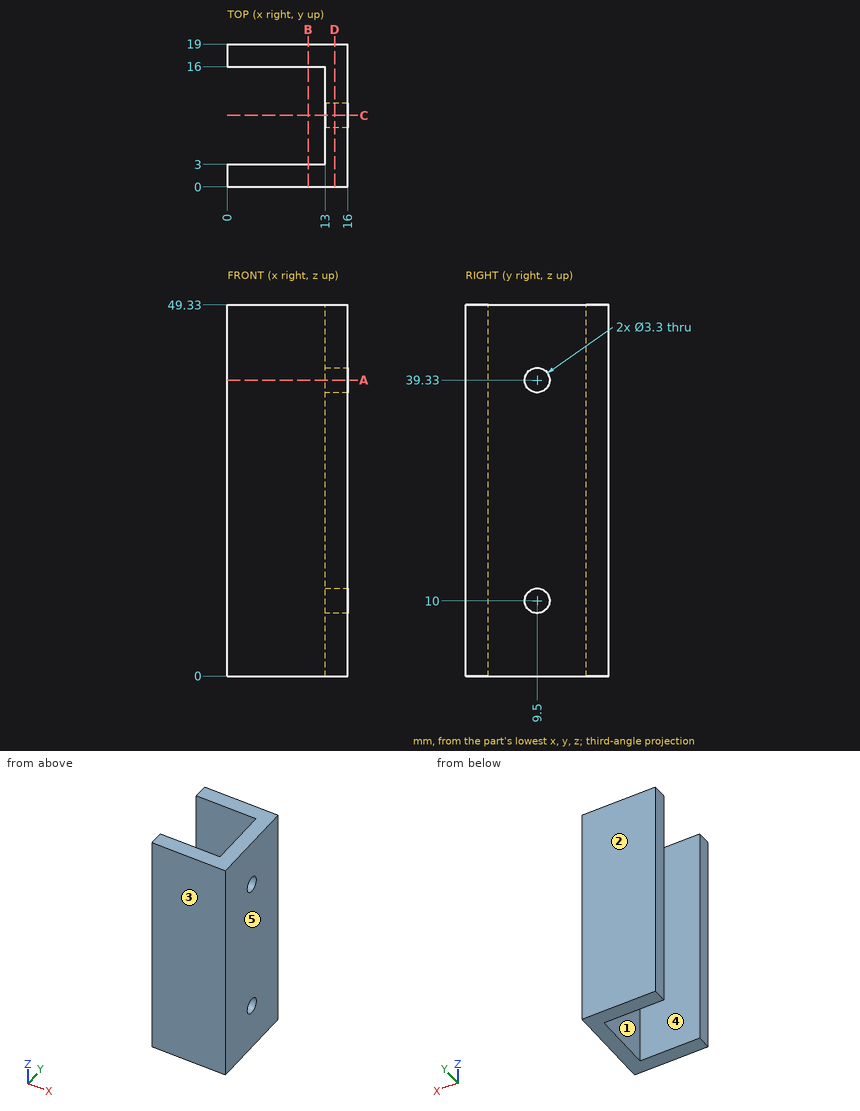
Can you work these out from the drawing? Everything is in mm from the part's minimum corner. A direction names the side the tool comes from. Round coordinates to 2 decimals unless told otherwise and drop trailing zeros. Order: outer loops, then holes, each group sorted by start corner. A loop starts at its lowest first (then second) coordinate and runs counter-clockwise, first axis right, second up. Notation, with made-up numbers: M 27,-37 L 59,-37 A27 cw 59,-15 Z; hole C -25,58.5 d11. An arc over 180 degrees is marked long. One line per question, with ' | ' between items.
1) I want a section at D-D, the plane x = 14.25. Write out the boundary of the cut face in (y, z).
Working result:
outline: M 0,0 L 19,0 L 19,49.33 L 0,49.33 Z; hole C 9.5,10 d3.3; hole C 9.5,39.33 d3.3
2) For the marked faces 4 and 5, which set-ups out of +Z, -Z, +X, -X, +Y, -Y let a thin tool reach every point of the face, with its end or its side?
Working result:
face 4: +Z, -Z, -X | face 5: +Z, -Z, +X, +Y, -Y
3) For pin 1 Ø2.5 at (y, z) = (9.5, 39.33) entering from +X, with a flat end and sliding along its axis, tell me the tip position at first contact or that it passes through.
Working result:
pin 1: through
4) I want a section at C-C, the plane y = 9.5. Write out the boundary of the cut face in (x, z).
Working result:
outline: M 13,0 L 16,0 L 16,8.35 L 13,8.35 Z; M 13,11.65 L 16,11.65 L 16,37.68 L 13,37.68 Z; M 13,40.98 L 16,40.98 L 16,49.33 L 13,49.33 Z
5) If we mould it in two halves opening along Y, with no side actions, what happens to the marked faces 1, 2 and 3? For each: +Y half, -Y half, draft (parallel to the pull), parting line (faces both ways), or undercut.
Working result:
face 1: undercut | face 2: +Y half | face 3: -Y half
6) I want a section at B-B, the plane x = 10.75. Write out the boundary of the cut face in (y, z).
Working result:
outline: M 0,0 L 3,0 L 3,49.33 L 0,49.33 Z; M 16,0 L 19,0 L 19,49.33 L 16,49.33 Z
7) I need wall thicknesses on line 1 along Y through (x, z) = (9.75, 3); line 2 along Y through (x, z) = (14.65, 10); line 3 along X through (y, z) = (7.5, 33.5). Which ranges of each line are inside material? Lowest first, please.
Working result:
line 1: 0 to 3, 16 to 19 | line 2: 0 to 7.85, 11.15 to 19 | line 3: 13 to 16
8) I want a section at A-A, the plane z = 39.33. Write out the boundary of the cut face in (x, y), then the cut area to 3 significant figures.
Working result:
outline: M 0,0 L 16,0 L 16,7.85 L 13,7.85 L 13,3 L 0,3 Z; M 0,16 L 13,16 L 13,11.15 L 16,11.15 L 16,19 L 0,19 Z | area: 125 mm²
